```python
from build123d import *

# Parameters (mm, degrees)
SKETCH1_W           = 44.45
SKETCH1_H           = 63.5
SKETCH1_R           = 1.27
BOSS_EXTRUDE1_DEPTH = 6.35
SKETCH2_W           = 22.606
SKETCH2_H           = 42.672
CUT_EXTRUDE1_DEPTH  = 7.35
SKETCH3_W           = 3.175
SKETCH3_H           = 16.248427567
CUT_EXTRUDE2_DEPTH  = 7.35
FILLET1_R           = 6.35


with BuildPart() as part:
    # Sketch1 → Boss-Extrude1 (new body)
    with BuildSketch(Plane.XY):
        Rectangle(SKETCH1_W, SKETCH1_H)
        with Locations((-4.999806813, 25.351447061)):
            Circle(SKETCH1_R, mode=Mode.SUBTRACT)
        with Locations((4.999565199, 25.350804136)):
            Circle(SKETCH1_R, mode=Mode.SUBTRACT)
        with Locations((-5.000419542, -25.352292054)):
            Circle(SKETCH1_R, mode=Mode.SUBTRACT)
        with Locations((4.999806813, -25.351447061)):
            Circle(SKETCH1_R, mode=Mode.SUBTRACT)
    extrude(amount=BOSS_EXTRUDE1_DEPTH)

    # Sketch2 → Cut-Extrude1 (cut, through all)
    with BuildSketch(Plane.XY.offset(6.35)):
        Rectangle(SKETCH2_W, SKETCH2_H)
    extrude(amount=-CUT_EXTRUDE1_DEPTH, mode=Mode.SUBTRACT)

    # Sketch3 → Cut-Extrude2 (cut, through all)
    with BuildSketch(Plane.XY.offset(6.35)):
        with Locations((0, 27.215647874)):
            Rectangle(SKETCH3_W, SKETCH3_H)
    extrude(amount=-CUT_EXTRUDE2_DEPTH, mode=Mode.SUBTRACT)

    # Fillet1
    fillet1_edges = [part.edges().sort_by_distance(p)[0] for p in [
        (-22.225, 31.75, 3.175),
        (22.225, 31.75, 3.175),
        (22.225, -31.75, 3.175),
        (-22.225, -31.75, 3.175),
    ]]
    fillet(fillet1_edges, radius=FILLET1_R)


solid = part.part
```
Check sheet for the modelled part. Datum: model origin and axes. Units: mm. A direction names the side the tool comes from. Coordinates: 2 decimals unless noted, no trailing zeros. Loops run counter-clockwise (first coordinate to the right, second up) from the corner with the lowest first, then second, coordinate; pieces in that order, holes last.
1) Sectioned sample at C-C (z = 4.25). Count the separate pieces of the cut face and the enclosed holes in it, and give its area (3 significant figures).
2) Access from +Z, -Z, +X, -X, +Y, -Y to the whole of each face (thin tool, end or side, straight path). Record for faces 4 (the face through (-11.303, 0, 3)), 5 (the face through (-1.588, 26, 3)), 6 (the face through (0, -31.75, 3)).
3) Release check for a two-part mould opening along Y. For faces 1 (the face through (-7, 21.336, 3)), 2 (the face through (-20.414, 29.84, 3.219)), 3 (the face through (-20.414, -29.84, 3.219)) record: released by +Y, released by -Y, zero draft, split by the parting line, or undercut.
4) Sectioned sample at A-A (y = 0). Record the boundary of the cut face in (x, z) (3 decimals).
5) Sectioned sample at B-B (x = -8). Record the boundary of the cut face in (y, z), and give its area (3 significant figures).
6) Gauge pin test, flat ends, axial feed: pin 1 (2 mm diameter, centred on x = -5, y = 25.35, fed in from +Z); pin 2 (12 mm diameter, centred on x = 14, y = 21, fed in from -Z); pin 3 (1.9 mm diameter, centred on x = 0, z = 3, fed in from +Y). Record the tip position at first contact, or that the pin passes through.
7) Material ranges on probe 1 along X at (y, z) = (16, 5.5) (3 decimals); probe 2 along X at (y, z) = (22.5, 5.5) (1 decimal); probe 3 along Y at (x, z) = (-3, 2.75), recorded low to high.
8) Sectioned sample at D-D (x = 0.5). Record the boundary of the cut face in (y, z).
Check sheet entries:
1. separate pieces: 1
1. enclosed holes: 4
1. area: 1,770 mm2
2. face 4: +Z, -Z
2. face 5: +Z, -Z, +Y
2. face 6: +Z, -Z, +X, -X, -Y
3. face 1: undercut
3. face 2: released by +Y
3. face 3: released by -Y
4. outline: (-22.225, 0) - (-11.303, 0) - (-11.303, 6.35) - (-22.225, 6.35) - close; (11.303, 0) - (22.225, 0) - (22.225, 6.35) - (11.303, 6.35) - close
5. outline: (-31.75, 0) - (-21.34, 0) - (-21.34, 6.35) - (-31.75, 6.35) - close; (21.34, 0) - (31.75, 0) - (31.75, 6.35) - (21.34, 6.35) - close
5. area: 132 mm2
6. pin 1: passes through
6. pin 2: stops at z = 0
6. pin 3: stops at y = -21.34
7. probe 1: x = -22.225 to -11.303, 11.303 to 22.225
7. probe 2: x = -22.2 to -1.6, 1.6 to 22.2
7. probe 3: y = -31.75 to -21.34, 21.34 to 31.75
8. outline: (-31.75, 0) - (-21.34, 0) - (-21.34, 6.35) - (-31.75, 6.35) - close
